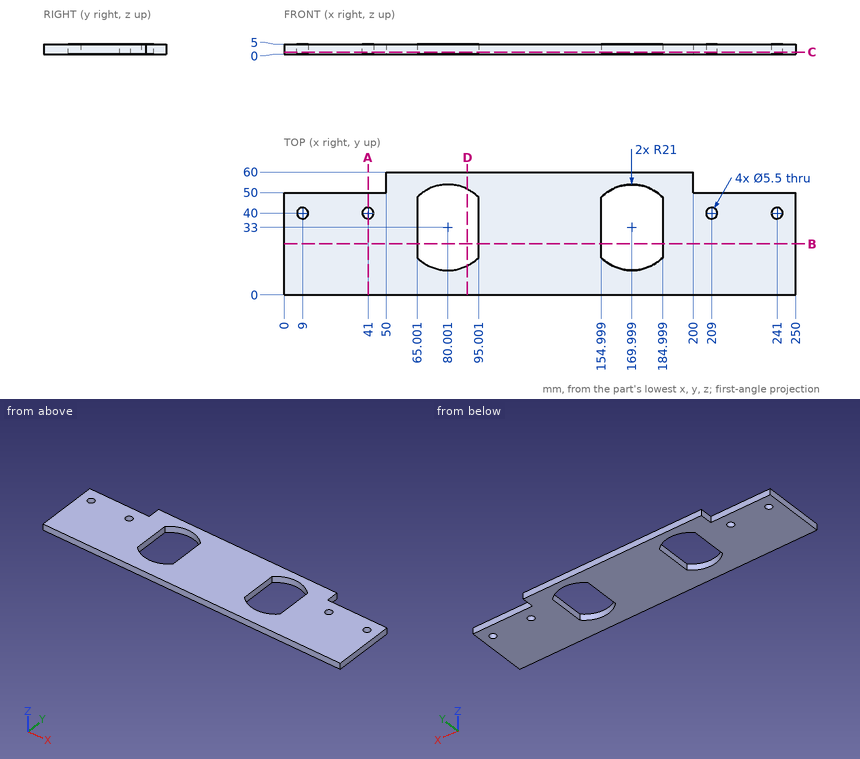
Verification items for this drawing (mm, ordinates from the low corner). Coordinates: 2 decimals unless noted, no trailing zeros. Loops run counter-clockwise (first coordinate to the right, second up) from the corner with the lowest first, then second, coordinate; pieces in that order, holes last. Notation, with made-up numbers: (8.25, -25) -> (30.25, -25) arc R16 cw to (30.25, -5) -> close; hole circle Ø11 at (-8.5, 10). An arc over 180 degrees is marked (long way). Answer in a Markdown table with one row per item. Add a question column.
1. Depth check by flat-ended pin: P1, Ø2.5, axis at x = 24, z = 1.5, coming from the +Y side; P2, Ø1.5, axis at y = 52.5, z = 3, coming from the +X side. Enter the tip coordinate at first touch or a pass-through.
2. Section check C-C, the plane z = 1. Enter the section's corners in (x, y).
3. Material ranges on probe 1 along X at (y, z) = (26, 4.75); probe 2 along Y at (x, z) = (81, 2.85); probe 3 along Y at (x, z) = (241, 2.5), recorded low to high. Write a range as [from, to].
4. Section check A-A, the plane x = 41. Enter the section's corners in (y, z).
5. Section check D-D, the plane x = 89.5. Enter the section's corners in (y, z).
6. Section check B-B, the plane y = 25. Enter the section's corners in (x, z).
Derived:
| question | item | result |
|---|---|---|
| 1 | P1 | stops at y = 50 |
| 1 | P2 | stops at x = 200 |
| 2 | outline | (0, 0) -> (250, 0) -> (250, 50) -> (200, 50) -> (200, 60) -> (50, 60) -> (50, 50) -> (0, 50) -> close; hole circle Ø5.5 at (9, 40); hole circle Ø5.5 at (41, 40); hole (65, 18.3) arc R21 ccw to (95, 18.3) -> (95, 47.7) arc R21 ccw to (65, 47.7) -> close; hole (155, 18.3) arc R21 ccw to (185, 18.3) -> (185, 47.7) arc R21 ccw to (155, 47.7) -> close; hole circle Ø5.5 at (209, 40); hole circle Ø5.5 at (241, 40) |
| 3 | probe 1 | x = [0, 65], [95, 155], [185, 250] |
| 3 | probe 2 | y = [0, 12.02], [53.98, 60] |
| 3 | probe 3 | y = [0, 37.25], [42.75, 50] |
| 4 | outline | (0, 0) -> (37.25, 0) -> (37.25, 5) -> (0, 5) -> close; (42.75, 0) -> (50, 0) -> (50, 5) -> (42.75, 5) -> close |
| 5 | outline | (0, 0) -> (14.27, 0) -> (14.27, 5) -> (0, 5) -> close; (51.73, 0) -> (60, 0) -> (60, 5) -> (51.73, 5) -> close |
| 6 | outline | (0, 0) -> (65, 0) -> (65, 5) -> (0, 5) -> close; (95, 0) -> (155, 0) -> (155, 5) -> (95, 5) -> close; (185, 0) -> (250, 0) -> (250, 5) -> (185, 5) -> close |
